Verification items for the finished model (mm, model axes). A direction names the side the tool comes from. Give positions to 0.01 mm unless a question says otherwise; leave off trailing zeros. Write each loop counter-clockwise with the first axis right and the second up, starting at its lowest first coordinate (ties: lowest second). Pieces come first, ordered by that corner, then holes.
from build123d import *

# Parameters (mm, degrees)
SKIZZE1_R                       = 12
SKIZZE1_R_2                     = 10.05
AUFSATZ_LINEAR_AUSTRAGEN1_DEPTH = 1.8
SKIZZE2_W                       = 4.4
SKIZZE2_H                       = 12.957963354
AUFSATZ_LINEAR_AUSTRAGEN2_DEPTH = 1
VERRUNDUNG1_R                   = 5
VERRUNDUNG2_R                   = 1
AUFSATZ_LINEAR_AUSTRAGEN3_DEPTH = 1.8


with BuildPart() as part:
    # Skizze1 → Aufsatz-Linear austragen1 (new body)
    with BuildSketch(Plane.XY):
        Circle(SKIZZE1_R)
        Circle(SKIZZE1_R_2, mode=Mode.SUBTRACT)
    extrude(amount=AUFSATZ_LINEAR_AUSTRAGEN1_DEPTH)

    # Skizze2 → Aufsatz-Linear austragen2 (add)
    with BuildSketch(Plane.XY.offset(1.8)):
        with Locations((1.8, -16.521018323)):
            Rectangle(SKIZZE2_W, SKIZZE2_H)
    extrude(amount=-AUFSATZ_LINEAR_AUSTRAGEN2_DEPTH)

    # Verrundung1
    verrundung1_edges = [part.edges().sort_by_distance(p)[0] for p in [
        (-0.4, -11.99333148, 1.3),
        (4, -11.313708499, 1.3),
    ]]
    fillet(verrundung1_edges, radius=VERRUNDUNG1_R)

    # Verrundung2
    verrundung2_edges = [part.edges().sort_by_distance(p)[0] for p in [
        (-0.4, -23, 1.3),
        (4, -23, 1.3),
    ]]
    fillet(verrundung2_edges, radius=VERRUNDUNG2_R)

    # Skizze1<3> → Aufsatz-Linear austragen3 (add)
    with BuildSketch(Plane.XY):
        with BuildLine():
            Line((-8.685254038, -5.056566256), (-8.685254038, 5.056566256))
            ThreePointArc((-8.685254038, 5.056566256), (-10.05, 0), (-8.685254038, -5.056566256))
        make_face()
        with BuildLine():
            ThreePointArc((10.05, 0), (9.702816681, 2.618749408), (8.685254038, 5.056566256))
            Line((8.685254038, 5.056566256), (8.685254038, -5.056566256))
            ThreePointArc((8.685254038, -5.056566256), (9.702816681, -2.618749408), (10.05, 0))
        make_face()
    extrude(amount=AUFSATZ_LINEAR_AUSTRAGEN3_DEPTH)


solid = part.part
Item 1: Release check for a two-part mould opening along X. For faces 1 (the face through (4, -18, 1)), 2 (the face through (0.15, 10.05, 0.89)), 3 (the face through (9, 0, 0)) record: released by +X, released by -X, zero draft, split by the parting line, or undercut.
Answer key:
face 1: released by +X
face 2: undercut
face 3: zero draft
Item 2: Sectioned sample at D-D on x = 7.5. Record the cut outline in (y, z).
Answer key:
outline: (-9.37, 0) - (-6.69, 0) - (-6.69, 1.8) - (-9.37, 1.8) - close; (6.69, 0) - (9.37, 0) - (9.37, 1.8) - (6.69, 1.8) - close
Item 3: Sectioned sample at B-B on y = 0. Record the cut outline in (x, z).
Answer key:
outline: (-12, 0) - (-8.69, 0) - (-8.69, 1.8) - (-12, 1.8) - close; (8.69, 0) - (12, 0) - (12, 1.8) - (8.69, 1.8) - close
Item 4: Depth check by flat-ended pin: pin 1 (0.8 mm diameter, centred on y = -18.5, z = 1, fed in from -X); pin 2 (0.9 mm diameter, centred on y = -2.5, z = 0.5, fed in from +X); pin 3 (5 mm diameter, centred on x = -1, y = -16, fed in from -Z). Enter the tip coordinate at first touch or a pass-through.
Answer key:
pin 1: stops at x = -0.4
pin 2: stops at x = 11.82
pin 3: stops at z = 0.8
Item 5: Sectioned sample at C-C on z = 1.4. Record the cut outline in (x, y).
Answer key:
outline: (-3.81, -11.38) arc R5 cw to (-0.4, -16.12) - (-0.4, -22) arc R1 ccw to (0.6, -23) - (3, -23) arc R1 ccw to (4, -22) - (4, -14.42) arc R5 cw to (6.35, -10.18) arc R12 ccw (long way) to start; hole (-8.69, -5.06) arc R10.05 ccw to (-0.4, -10.04) - (0.4, -10.04) arc R10.05 ccw to (8.69, -5.06) - (8.69, 5.06) arc R10.05 ccw to (-8.69, 5.06) - close
Item 6: Scan lines: line 1 along Y through (x, z) = (0.25, 0.1); line 2 along X through (y, z) = (4.5, 1.35); line 3 along Y through (x, z) = (-5.5, 1.15). Record each from-to range of solid material in increasing order.
Answer key:
line 1: y = -12 to -10.05, 10.05 to 12
line 2: x = -11.12 to -8.69, 8.69 to 11.12
line 3: y = -10.67 to -8.41, 8.41 to 10.67
Item 7: Set-up check for faces 4 (the face through (3.715, -22.699, 1.293)), 5 (the face through (-0.4, -19, 1)), 6 (the face through (-8.685, 0, 1)): record each of +Z, -Z, +X, -X, +Y, -Y from which the full face is reachable in a straight line by a thin tool's end or side.
Answer key:
face 4: +Z, -Z, +X, -Y
face 5: +Z, -Z, -X, -Y
face 6: +Z, -Z
